Source: CAD feature listing. Evaluate the final solid. Frame: model axes, mm. Face numbers are marked on the shaded views. Round coordinates to 2 decimals unless told otherwise and drop trailing zeros. Order: outer loops, then holes, each group sorted by start corner. A loop starts at its lowest first (then second) coordinate and runs counter-clockwise, first axis right, second up. Notation, with made-up numbers: (79.25, 56.25) - (93.25, 56.25) arc R19 ccw to (93.25, 78.25) - close; hole circle Ø9 at (-5, 38.5). An arc over 180 degrees is marked (long way). Return JSON: item names as keys, results as strings. Group by question number.
1) Contact query for flat-ended pins moving along their axis: P1, Ø0.6, axis at x = -30.5, z = 0, coming from the -Y side; P2, Ø17, axis at x = 16, z = 11, coming from the +Y side. Output: stop coordinate, or through.
2) Section B-B, the plane z = -20. Return loops of the section in (x, y), plus the area to 4 significant figures.
3) Section A-A, the plane x = -17. Return loops of the section in (y, z).
4) Section D-D, the plane z = 0. Return loops of the section in (x, y), plus the area to 4 significant figures.
5) Mould query, pull axis Z, two halves, no side actions, for the marked faces 1, 2 and 3. Classes: pulls with the +Z half, pulls with the -Z half, needs draft (parallel to the pull), parting line crosses it, or undercut.
6) Section C-C, the plane x = 30.75. Return loops of the section in (y, z), plus the area to 3 significant figures.
7) Ray query, line 1 (X direction, y = 0.45, z = 0); line 2 (Y direction, x = 6.5, z = 12.5); line 3 (Y direction, x = 26, z = 16.5). Return the intervals inside material, ascending. Write a range as from..to.
```python
from build123d import *

# Parameters (mm, degrees)
BOSS_EXTRUDE1_DEPTH      = 13
CUT_EXTRUDE1_DEPTH       = 0.1
SKETCH3_W                = 50.5
SKETCH3_H                = 40.4
BOSS_EXTRUDE2_DEPTH      = 0.1
SKETCH4_R                = 2
BOSS_EXTRUDE3_DEPTH      = 1
BOSS_EXTRUDE3_DEPTH_BACK = 1
SKETCH5_R                = 4
BOSS_EXTRUDE4_DEPTH      = 2
SKETCH6_R                = 1
CUT_EXTRUDE3_DEPTH       = 2


with BuildPart() as part:
    # Sketch1 → Boss-Extrude1 (new body)
    with BuildSketch(Plane(origin=(0, 0, 0), x_dir=(1, 0, 0), z_dir=(0, 1, 0))):
        with BuildLine():
            Line((32.25, 28.7), (-32.25, 28.7))
            ThreePointArc((-32.25, 28.7), (-35.078427125, 27.528427125), (-36.25, 24.7))
            Line((-36.25, 24.7), (-36.25, -24.7))
            ThreePointArc((-36.25, -24.7), (-35.078427125, -27.528427125), (-32.25, -28.7))
            Line((-32.25, -28.7), (32.25, -28.7))
            ThreePointArc((32.25, -28.7), (35.078427125, -27.528427125), (36.25, -24.7))
            Line((36.25, -24.7), (36.25, 24.7))
            ThreePointArc((36.25, 24.7), (35.078427125, 27.528427125), (32.25, 28.7))
        make_face()
    extrude(amount=BOSS_EXTRUDE1_DEPTH)

    # Sketch2 → Cut-Extrude1 (cut)
    with BuildSketch(Plane(origin=(0, 13, 0), x_dir=(1, 0, 0), z_dir=(0, 1, 0))):
        with BuildLine():
            Line((-27.25, -26.75), (-27.25, -24.65))
            ThreePointArc((-27.25, -24.65), (-27.191421356, -24.508578644), (-27.05, -24.45))
            Line((-27.05, -24.45), (-26.95, -24.45))
            ThreePointArc((-26.95, -24.45), (-26.808578644, -24.508578644), (-26.75, -24.65))
            Line((-26.75, -24.65), (-26.75, -26.75))
            ThreePointArc((-26.75, -26.75), (-26.808578644, -26.891421356), (-26.95, -26.95))
            Line((-26.95, -26.95), (-27.05, -26.95))
            ThreePointArc((-27.05, -26.95), (-27.191421356, -26.891421356), (-27.25, -26.75))
        make_face()
        with BuildLine():
            Line((-32.25, -22.7), (32.25, -22.7))
            ThreePointArc((32.25, -22.7), (34.371320344, -21.821320344), (35.25, -19.7))
            Line((35.25, -19.7), (35.25, 24.7))
            ThreePointArc((35.25, 24.7), (34.371320344, 26.821320344), (32.25, 27.7))
            Line((32.25, 27.7), (-32.25, 27.7))
            ThreePointArc((-32.25, 27.7), (-34.371320344, 26.821320344), (-35.25, 24.7))
            Line((-35.25, 24.7), (-35.25, -19.7))
            ThreePointArc((-35.25, -19.7), (-34.371320344, -21.821320344), (-32.25, -22.7))
        make_face()
        with BuildLine():
            Line((-28.25, -26.75), (-28.25, -24.65))
            ThreePointArc((-28.25, -24.65), (-28.191421356, -24.508578644), (-28.05, -24.45))
            Line((-28.05, -24.45), (-27.95, -24.45))
            ThreePointArc((-27.95, -24.45), (-27.808578644, -24.508578644), (-27.75, -24.65))
            Line((-27.75, -24.65), (-27.75, -26.75))
            ThreePointArc((-27.75, -26.75), (-27.808578644, -26.891421356), (-27.95, -26.95))
            Line((-27.95, -26.95), (-28.05, -26.95))
            ThreePointArc((-28.05, -26.95), (-28.191421356, -26.891421356), (-28.25, -26.75))
        make_face()
        with BuildLine():
            Line((-26.25, -26.75), (-26.25, -24.65))
            ThreePointArc((-26.25, -24.65), (-26.191421356, -24.508578644), (-26.05, -24.45))
            Line((-26.05, -24.45), (-25.95, -24.45))
            ThreePointArc((-25.95, -24.45), (-25.808578644, -24.508578644), (-25.75, -24.65))
            Line((-25.75, -24.65), (-25.75, -26.75))
            ThreePointArc((-25.75, -26.75), (-25.808578644, -26.891421356), (-25.95, -26.95))
            Line((-25.95, -26.95), (-26.05, -26.95))
            ThreePointArc((-26.05, -26.95), (-26.191421356, -26.891421356), (-26.25, -26.75))
        make_face()
        with BuildLine():
            Line((-25.25, -26.75), (-25.25, -24.65))
            ThreePointArc((-25.25, -24.65), (-25.191421356, -24.508578644), (-25.05, -24.45))
            Line((-25.05, -24.45), (-24.95, -24.45))
            ThreePointArc((-24.95, -24.45), (-24.808578644, -24.508578644), (-24.75, -24.65))
            Line((-24.75, -24.65), (-24.75, -26.75))
            ThreePointArc((-24.75, -26.75), (-24.808578644, -26.891421356), (-24.95, -26.95))
            Line((-24.95, -26.95), (-25.05, -26.95))
            ThreePointArc((-25.05, -26.95), (-25.191421356, -26.891421356), (-25.25, -26.75))
        make_face()
    extrude(amount=-CUT_EXTRUDE1_DEPTH, mode=Mode.SUBTRACT)

    # Sketch3 → Boss-Extrude2 (add)
    with BuildSketch(Plane(origin=(0, 12.9, 0), x_dir=(1, 0, 0), z_dir=(0, 1, 0))):
        with Locations((0, 2.5)):
            Rectangle(SKETCH3_W, SKETCH3_H)
    extrude(amount=BOSS_EXTRUDE2_DEPTH)

    # Sketch4 → Boss-Extrude3 (add, two sides)
    with BuildSketch(Plane(origin=(0, 13, 0), x_dir=(1, 0, 0), z_dir=(0, 1, 0))) as boss_extrude3_sk:
        with Locations(Location((27.75, -21.7, 0), (0, 0, 270))):  # turned: the seam where the file's is
            Circle(SKETCH4_R)
    extrude(amount=BOSS_EXTRUDE3_DEPTH)
    extrude(boss_extrude3_sk.sketch, amount=-BOSS_EXTRUDE3_DEPTH_BACK)

    # Sketch5 → Boss-Extrude4 (add)
    with BuildSketch(Plane(origin=(0, 14, 0), x_dir=(1, 0, 0), z_dir=(0, 1, 0))):
        with Locations(Location((27.75, -21.7, 0), (0, 0, 270))):  # turned: the seam where the file's is
            Circle(SKETCH5_R)
    extrude(amount=BOSS_EXTRUDE4_DEPTH)

    # Sketch6 → Cut-Extrude3 (cut)
    with BuildSketch(Plane.XZ):
        with Locations(Location((30.75, 0, 0), (0, 0, 270))):  # turned: the seam where the file's is
            Circle(SKETCH6_R)
        with Locations(Location((-30.75, 0, 0), (0, 0, 270))):  # turned: the seam where the file's is
            Circle(SKETCH6_R)
    extrude(amount=-CUT_EXTRUDE3_DEPTH, mode=Mode.SUBTRACT)


solid = part.part
```
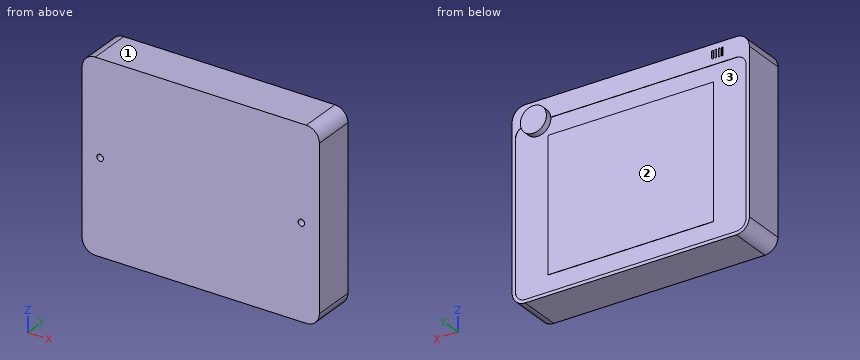
Geometry check:
{
 "1": {"P1": "y = 2", "P2": "y = 13"},
 "2": {"outline": "(-36.25, 0) - (36.25, 0) - (36.25, 13) - (35.25, 13) - (35.25, 12.9) - (25.25, 12.9) - (25.25, 13) - (-25.25, 13) - (-25.25, 12.9) - (-35.25, 12.9) - (-35.25, 13) - (-36.25, 13) - close", "area": "940.5 mm2"},
 "3": {"outline": "(0, -28.7) - (13, -28.7) - (13, -27.7) - (12.9, -27.7) - (12.9, -22.7) - (13, -22.7) - (13, 17.7) - (12.9, 17.7) - (12.9, 22.7) - (13, 22.7) - (13, 28.7) - (0, 28.7) - close"},
 "4": {"outline": "(-36.25, 0) - (-31.75, 0) - (-31.75, 2) - (-29.75, 2) - (-29.75, 0) - (29.75, 0) - (29.75, 2) - (31.75, 2) - (31.75, 0) - (36.25, 0) - (36.25, 13) - (35.25, 13) - (35.25, 12.9) - (25.25, 12.9) - (25.25, 13) - (-25.25, 13) - (-25.25, 12.9) - (-35.25, 12.9) - (-35.25, 13) - (-36.25, 13) - close", "area": "932.5 mm2"},
 "5": {"face 1": "pulls with the +Z half", "face 2": "needs draft", "face 3": "undercut"},
 "6": {"outline": "(0, -28.7) - (13, -28.7) - (13, -27.7) - (12.9, -27.7) - (12.9, 22.7) - (13, 22.7) - (13, 28.7) - (0, 28.7) - (0, 1) - (2, 1) - (2, -1) - (0, -1) - close; (14, 19.05) - (16, 19.05) - (16, 24.35) - (14, 24.35) - close", "area": "748 mm2"},
 "7": {"line 1": "-36.25..-31.75, -29.75..29.75, 31.75..36.25", "line 2": "0..13", "line 3": "0..12.9"}
}
